```python
from build123d import *

# Parameters (mm, degrees)
F0_W     = 50
F0_H     = 120
F1_DEPTH = 4
F2_W     = 4
F2_H     = 20
F2_H_2   = 10
F3_DEPTH = 4
F5_D     = 3.3


with BuildPart() as f1:
    # F0 (on Front) → F1 (new body)
    with BuildSketch(Plane.XZ):
        Rectangle(F0_W, F0_H)
        Polygon((-21.4033009983, -30.4732918523), (-20.0139842574, -29.0346122516), (-12.820586254, -35.9811959562), (-14.2099029949, -37.4198755569), (-15.5992197358, -38.8585551576), (-22.7926177392, -31.911971453), align=None, mode=Mode.SUBTRACT)
        Polygon((-1.2124237291, -52.7517225667), (-8.4058217325, -45.8051388622), (-7.0165049915, -44.3664592615), (-5.6271882506, -42.9277796608), (1.5662097528, -49.8743633654), (0.1768930119, -51.3130429661), align=None, mode=Mode.SUBTRACT)
        Polygon((5.6271882506, -0.9277796608), (7.0165049915, -2.3664592615), (8.4058217325, -3.8051388622), (1.2124237291, -10.7517225667), (-0.1768930119, -9.3130429661), (-1.5662097528, -7.8743633654), align=None, mode=Mode.SUBTRACT)
        Polygon((-22.7926177392, 52.088028547), (-21.4033009983, 53.5267081477), (-20.0139842574, 54.9653877484), (-12.820586254, 48.0188040438), (-14.2099029949, 46.5801244431), (-15.5992197358, 45.1414448424), align=None, mode=Mode.SUBTRACT)
        Polygon((-8.4058217325, 38.1948611378), (-7.0165049915, 39.6335407385), (-5.6271882506, 41.0722203392), (1.5662097528, 34.1256366346), (0.1768930119, 32.6869570339), (-1.2124237291, 31.2482774333), align=None, mode=Mode.SUBTRACT)
        Polygon((20.0139842574, 12.9653877484), (21.4033009983, 11.5267081477), (22.7926177392, 10.088028547), (15.5992197358, 3.1414448424), (14.2099029949, 4.5801244431), (12.820586254, 6.0188040438), align=None, mode=Mode.SUBTRACT)
    extrude(amount=F1_DEPTH)

    # F2 (on face) → F3 (join)
    with BuildSketch(Plane.XZ.offset(4)):
        with Locations((-27, 40)):
            Rectangle(F2_W, F2_H)
        with Locations((-27, -5)):
            Rectangle(F2_W, F2_H_2)
        with Locations((-27, 5)):
            Rectangle(F2_W, F2_H_2)
        with Locations((-27, -40)):
            Rectangle(F2_W, F2_H)
        with Locations((27, 5)):
            Rectangle(F2_W, F2_H_2)
        with Locations((27, -5)):
            Rectangle(F2_W, F2_H_2)
        with Locations((27, 40)):
            Rectangle(F2_W, F2_H)
        with Locations((27, -40)):
            Rectangle(F2_W, F2_H)
    extrude(amount=-F3_DEPTH)

    # F5 (through all)
    with Locations(Plane.XZ.offset(4)):
        with Locations((-18, 0), (18, 0)):
            Hole(F5_D / 2)


solid = f1.part
```
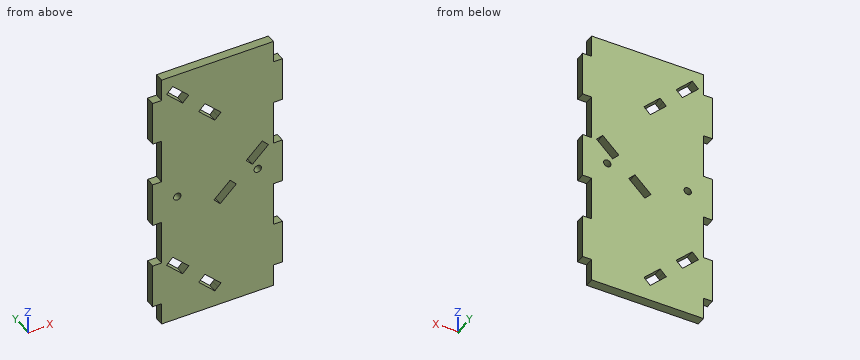
Part model, mm, in its own coordinate system. Give positions to 0.01 mm unless a question says otherwise; leave off trailing zeros. Write each loop counter-clockwise with the first axis right and the second up, starting at its lowest first coordinate (ties: lowest second). Pieces come first, ordered by that corner, then holes. Notation, with made-up numbers: (53, 23.5) -> (86, 23.5) arc R18 ccw to (86, 48.5) -> close; hole circle Ø11 at (51.25, -3). An arc over 180 degrees is marked (long way). Put each result on its own line as item: value. Start each with the question number.
Item 1: Cut at D-D (y = -2.25). State how many separate pieces and enclosed holes the cut face has, then the cut area to 3 significant figures.
Item 2: Wall check: L1, parallel to Z at x = -6, y = -0.55; L2, parallel to Z at x = -18, y = -1.6; L3, parallel to X at y = -1.95, z = -22.5. Give the ranges that are in metal, low to high. Write a range as [from, to].
Item 3: Cut at A-A (x = 18). List the corners of the cut face in (y, z), then the cut area to 3 significant figures.
Item 4: Cut at C-C (x = -18). List the corners of the cut face in (y, z).
Item 5: Cut at B-B (z = -5.5). List the corners of the cut face in (x, y), then the cut area to 3 significant figures.
Item 6: Pin check, flat tips, straight feed: pin 1 Ø1.2 at (y, z) = (-2, 20) entering from +X; pin 2 Ø2 at (x, y) = (27.5, -1) entering from +Z; pin 3 Ø3 at (x, z) = (-18, 0) entering from -Y; pin 4 Ø2 at (y, z) = (-3, 17.5) entering from -X. Stop position of each tip, or through.
Answer list:
1. separate pieces: 1
1. enclosed holes: 8
1. area: 6,220 mm2
2. L1: z = [-60, -48.13], [-43.31, 35.87], [40.69, 60]
2. L2: z = [-60, -36.54], [-30.98, -1.65], [1.65, 47.46], [53.02, 60]
2. L3: x = [-25, 25]
3. outline: (-4, -60) -> (0, -60) -> (0, -1.65) -> (-4, -1.65) -> close; (-4, 1.65) -> (0, 1.65) -> (0, 5.46) -> (-4, 5.46) -> close; (-4, 11.02) -> (0, 11.02) -> (0, 60) -> (-4, 60) -> close
3. area: 445 mm2
4. outline: (-4, -60) -> (0, -60) -> (0, -36.54) -> (-4, -36.54) -> close; (-4, -30.98) -> (0, -30.98) -> (0, -1.65) -> (-4, -1.65) -> close; (-4, 1.65) -> (0, 1.65) -> (0, 47.46) -> (-4, 47.46) -> close; (-4, 53.02) -> (0, 53.02) -> (0, 60) -> (-4, 60) -> close
5. outline: (-29, -4) -> (0.89, -4) -> (0.89, 0) -> (-29, 0) -> close; (6.65, -4) -> (29, -4) -> (29, 0) -> (6.65, 0) -> close
5. area: 209 mm2
6. pin 1: stops at x = 25
6. pin 2: stops at z = 50
6. pin 3: passes through
6. pin 4: stops at x = -25
